from build123d import *
from OCP.BRepAlgoAPI import BRepAlgoAPI_Cut
from OCP.TopTools import TopTools_ListOfShape

# Parameters (mm, degrees)
EXTRUDE_1_DEPTH     = 70
CUT_EXTRUDE_1_DEPTH = 20


with BuildPart() as part:
    # 草图2 → 凸台-拉伸1 (new body)
    with BuildSketch(Plane.XY):
        Polygon((-150.888329598, 26.350410604), (-100.888333902, 76.350410604), (-0.888333902, 76.350410604), (49.111670402, 26.350410604), (39.111670402, 26.350410604), (-0.888329598, 66.350410604), (-100.888329598, 66.350410604), (-140.888329598, 26.350410604), align=None)
    extrude(amount=EXTRUDE_1_DEPTH)


with BuildPart() as cut_extrude_1_tool:
    # 草图3 → 切除-拉伸1 (new body)
    with BuildSketch(Plane.XY.offset(70)):
        Polygon((-100.888333902, 76.350410604), (-0.888333902, 76.350410604), (24.111669326, 51.350411681), (14.111669326, 51.350411681), (-0.888329598, 66.350410604), (-100.888329598, 66.350410604), (-115.888330674, 51.350409528), (-125.888330674, 51.350409528), align=None)
    extrude(amount=-CUT_EXTRUDE_1_DEPTH)


with BuildPart() as part_1:
    add(part.part)

    # 切除-拉伸1: cut by cut_extrude_1_tool, with a tolerance
    cut_extrude_1_stock = TopTools_ListOfShape()
    cut_extrude_1_stock.Append(part_1.part.wrapped)
    cut_extrude_1_tools = TopTools_ListOfShape()
    cut_extrude_1_tools.Append(cut_extrude_1_tool.part.wrapped)
    cut_extrude_1_cut = BRepAlgoAPI_Cut()
    cut_extrude_1_cut.SetArguments(cut_extrude_1_stock)
    cut_extrude_1_cut.SetTools(cut_extrude_1_tools)
    cut_extrude_1_cut.SetFuzzyValue(0.00001)
    cut_extrude_1_cut.Build()
    add(Compound.cast(cut_extrude_1_cut.Shape()).solids(), mode=Mode.REPLACE)


solid = part_1.part
Design review of the part built by this model. Coordinates are the model's own, in mm. A direction names the side the tool comes from. Give positions to 0.01 mm unless a question says otherwise; leave off trailing zeros. Write each loop counter-clockwise with the first axis right and the second up, starting at its lowest first coordinate (ties: lowest second). Pieces come first, ordered by that corner, then holes. Notation, with made-up numbers: M -36,22.5 L -23,22.5 A15 cw -23,39.5 Z; hole C 79,2 d7. An arc over 180 degrees is marked long. Return JSON: item names as keys, results as strings. Group by question number.
Item 1: Take a section at D-D (x = -81). Give the boundary of the cut face in (y, z), plus the area to 3 significant figures.
Item 2: Wall thickness on line 1 along Y through (x, z) = (-6, 49.5); line 2 along Z through (x, y) = (-11, 72.5); line 3 along X through (y, z) = (39, 35.5): over which ranges is each line inside the solid? List them lowest first.
Item 3: Take a section at A-A (z = 37). Give the boundary of the cut face in (x, y).
Item 4: Take a section at C-C (y = 60.5). Give the boundary of the cut face in (x, z).
Item 5: Tool access review of faces 1 (the flat face through (-120.61, 46.63, 34.51)), 2 (the flat face through (23.76, 51.7, 26.73)), 3 (the flat face through (19, 51.35, 60)): name each direction out of +Z, -Z, +X, -X, +Y, -Y from which nothing blocks a thin tool from reaching the whole face with its end or side.
Item 6: Take a section at B-B (z = 59.5). Give the boundary of the cut face in (x, y).
Item 7: Clearance check with flat-ended pins moving along their axes: pin 1 Ø11 at (x, z) = (-122.5, 64.5) entering from +Y; pin 2 Ø2 at (y, z) = (54, 36) entering from +X; pin 3 Ø1 at (y, z) = (43.5, 57) entering from -X; pin 4 Ø3 at (x, y) = (-112.5, 61) entering from -Z. State where each tip first meets the part, or that it passes through.
Return value:
{
 "1": {"outline": "M 66.35,0 L 76.35,0 L 76.35,50 L 66.35,50 Z", "area": "500 mm2"},
 "2": {"line 1": "y = 66.35 to 76.35", "line 2": "z = 0 to 50", "line 3": "x = -138.24 to -128.24, 26.46 to 36.46"},
 "3": {"outline": "M -150.89,26.35 L -140.89,26.35 L -100.89,66.35 L -0.89,66.35 L 39.11,26.35 L 49.11,26.35 L -0.89,76.35 L -100.89,76.35 Z"},
 "4": {"outline": "M -116.74,0 L -106.74,0 L -106.74,50 L -116.74,50 Z; M 4.96,0 L 14.96,0 L 14.96,50 L 4.96,50 Z"},
 "5": {"face 1": "+Z, -Z, -Y", "face 2": "+Z, -Z, +X, +Y", "face 3": "+Z, +X, -X, +Y"},
 "6": {"outline": "M -150.89,26.35 L -140.89,26.35 L -115.89,51.35 L -125.89,51.35 Z; M 14.11,51.35 L 39.11,26.35 L 49.11,26.35 L 24.11,51.35 Z"},
 "7": {"pin 1": "stops at y = 51.35", "pin 2": "stops at x = 22.46", "pin 3": "stops at x = -134.24", "pin 4": "stops at z = 0"}
}
